```python
from build123d import *

# Parameters (mm, degrees)
SKETCH_R     = 1.375
SKETCH_R_2   = 3.5
PAD_DEPTH    = 8
SKETCH001_W  = 30
SKETCH001_H  = 5
POCKET_DEPTH = 98


with BuildPart() as part:
    # Sketch → Pad (new body)
    with BuildSketch(Plane.XY):
        Polygon((0, 0), (65, 0), (65, -30), (0, -30), (-33, -30), (-33, -35), (-73, -35), (-73, -22), (-33, -22), (0, -22), (0, -8), (-33, -8), (-73, -8), (-73, 5), (-33, 5), (-33, 0), align=None)
        with Locations((3.5, -3.5)):
            Circle(SKETCH_R, mode=Mode.SUBTRACT)
        with Locations((61.5, -3.5)):
            Circle(SKETCH_R, mode=Mode.SUBTRACT)
        with Locations((3.5, -26.5)):
            Circle(SKETCH_R, mode=Mode.SUBTRACT)
        with Locations((61.5, -26.5)):
            Circle(SKETCH_R, mode=Mode.SUBTRACT)
        with Locations((-68, 0)):
            Circle(SKETCH_R_2, mode=Mode.SUBTRACT)
        with Locations((-38, 0)):
            Circle(SKETCH_R_2, mode=Mode.SUBTRACT)
        with Locations((-68, -30)):
            Circle(SKETCH_R_2, mode=Mode.SUBTRACT)
        with Locations((-38, -30)):
            Circle(SKETCH_R_2, mode=Mode.SUBTRACT)
    extrude(amount=PAD_DEPTH)

    # Sketch001 → Pocket (cut)
    with BuildSketch(Plane.YZ.offset(65)):
        with Locations((-15, 5.5)):
            Rectangle(SKETCH001_W, SKETCH001_H)
    extrude(amount=-POCKET_DEPTH, mode=Mode.SUBTRACT)


solid = part.part
```
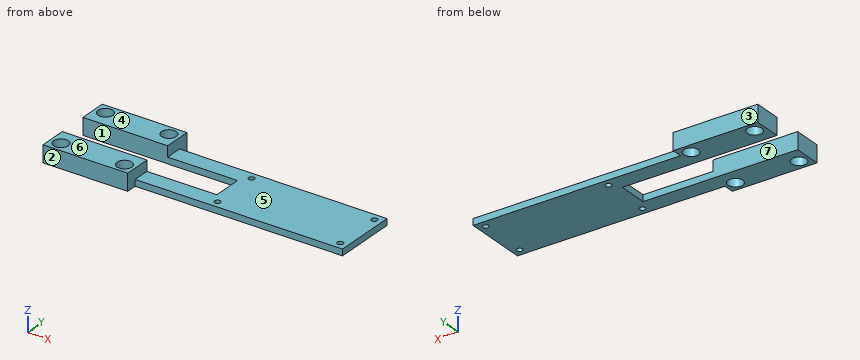
Design review of the part built by this model. Coordinates are the model's own, in mm. Face numbers are marked on the shaded views. A direction names the side the tool comes from. Round coordinates to 2 decimals unless told otherwise and drop trailing zeros. Order: outer loops, then holes, each group sorted by start corner. A loop starts at its lowest first (then second) coordinate and runs counter-clockwise, first axis right, second up. Notation, with made-up numbers: (72.25, 70.5) - (91.25, 70.5) arc R32 ccw to (91.25, 106.5) - close; hole circle Ø10 at (64.25, 1.5). An arc over 180 degrees is marked (long way). Return JSON: item names as keys, results as strings.
Q1. For pin 1 Ø6.5 at (x, y) = (-38, 0) entering from -Z; pin 2 Ø15 at (x, y) = (26, -20.5) entering from +Z; pin 3 Ø1.5 at (y, z) = (-14.5, 1) entering from -X; pin 4 Ø3.5 at (x, z) = (38, 1.5) entering from -Y, all flat-tipped, find the tip position at first contact; note any pin that passes through.
Computed values:
{"pin 1": "passes through", "pin 2": "stops at z = 3", "pin 3": "stops at x = 0", "pin 4": "stops at y = -30"}
Q2. The part is to be moulded in two halves that separate along Y. For the marked faces 1, 2, 3 and 4, say which applies: pulls with the +Y half, pulls with the -Y half, needs draft (parallel to the pull), parting line crosses it, or undercut.
Computed values:
{"face 1": "undercut", "face 2": "pulls with the -Y half", "face 3": "pulls with the +Y half", "face 4": "needs draft"}
Q3. Consider section A-A on z = 5.5. Write out the cut boundary in (x, y), plus the area to 3 significant figures.
Computed values:
{"outline": "(-73, -35) - (-33, -35) - (-33, -22) - (-73, -22) - close; (-73, -8) - (-33, -8) - (-33, 5) - (-73, 5) - close; hole circle Ø7 at (-68, -30); hole circle Ø7 at (-68, 0); hole circle Ø7 at (-38, -30); hole circle Ø7 at (-38, 0)", "area": "886 mm2"}
Q4. Machinability: for the marked faces 5, 6 and 7, which of the approach directions +Z, -Z, +X, -X, +Y, -Y give a long, thin tool a straight path to every point of the face, cutting with its end or side? Answer none if there is none.
Computed values:
{"face 5": "+Z, +X, +Y, -Y", "face 6": "+Z, +X, -X, +Y, -Y", "face 7": "+Z, -Z, -X"}
Q5. Consider section B-B on x = 61.5. Write out the cut boundary in (y, z) (3 decimals).
Computed values:
{"outline": "(-30, 0) - (-27.875, 0) - (-27.875, 3) - (-30, 3) - close; (-25.125, 0) - (-4.875, 0) - (-4.875, 3) - (-25.125, 3) - close; (-2.125, 0) - (0, 0) - (0, 3) - (-2.125, 3) - close"}
Q6. Consider section D-D on y = -9.5. Write out the cut boundary in (x, z), plus the area to 3 significant figures.
Computed values:
{"outline": "(0, 0) - (65, 0) - (65, 3) - (0, 3) - close", "area": "195 mm2"}
Q7. Consider section C-C on x = -68. Write out the cut boundary in (y, z).
Computed values:
{"outline": "(-35, 0) - (-33.5, 0) - (-33.5, 8) - (-35, 8) - close; (-26.5, 0) - (-22, 0) - (-22, 8) - (-26.5, 8) - close; (-8, 0) - (-3.5, 0) - (-3.5, 8) - (-8, 8) - close; (3.5, 0) - (5, 0) - (5, 8) - (3.5, 8) - close"}
Q8. Wall thickness on L1, parallel to Y at x = 3.5, z = 1.15 (3 decimals); L2, parallel to Y at x = -38, z = 3.5; L3, parallel to Y at x = -63.5, z = 5.25: over which ranges is each line inside the solid? List them lowest first. Write a range as [from, to].
Computed values:
{"L1": "y = [-30, -27.875], [-25.125, -4.875], [-2.125, 0]", "L2": "y = [-35, -33.5], [-26.5, -22], [-8, -3.5], [3.5, 5]", "L3": "y = [-35, -22], [-8, 5]"}
